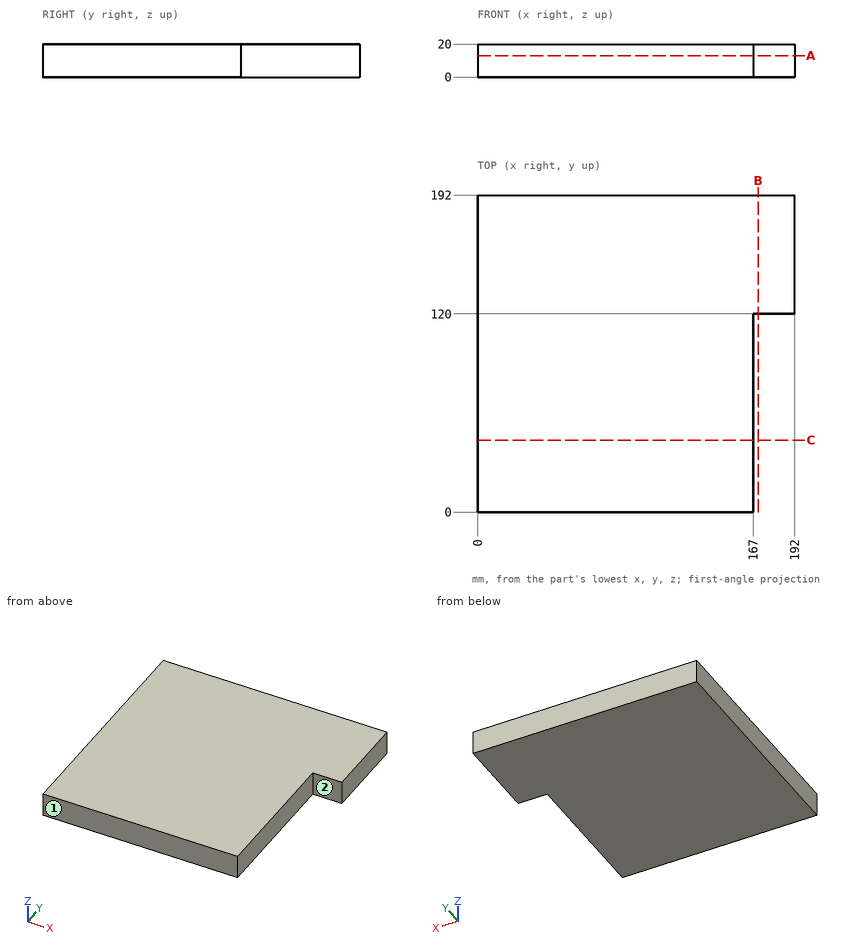
Geometry check sheet. Reference: drawing and pictorial views, mm from the part's lowest x, y, z. A direction names the side the tool comes from. Coordinates: 2 decimals unless noted, no trailing zeros. Loops run counter-clockwise (first coordinate to the right, second up) from the corner with the lowest first, then second, coordinate; pieces in that order, holes last.
1) Sectioned sample at A-A (z = 13). Record the boundary of the cut face in (x, y).
2) Gauge pin test, flat ends, axial feed: pin 1 (4 mm diameter, centred on y = 46.5, z = 8.5, fed in from -X); pin 2 (8 mm diameter, centred on y = 51.5, z = 17, fed in from +X). Record the tip position at first contact, or that the pin passes through.
3) Sectioned sample at C-C (y = 43.5). Record the boundary of the cut face in (x, z).
4) Sectioned sample at B-B (x = 170). Record the boundary of the cut face in (y, z), and give its area (3 significant figures).
5) Access from +Z, -Z, +X, -X, +Y, -Y to the whole of each face (thin tool, end or side, straight path). Record for the marked faces 1 and 2.
6) Material ranges on probe 1 along X at (y, z) = (106, 2), recorded low to high.
Check sheet entries:
1. outline: (0, 0) - (167, 0) - (167, 120) - (192, 120) - (192, 192) - (0, 192) - close
2. pin 1: stops at x = 0
2. pin 2: stops at x = 167
3. outline: (0, 0) - (167, 0) - (167, 20) - (0, 20) - close
4. outline: (120, 0) - (192, 0) - (192, 20) - (120, 20) - close
4. area: 1,440 mm2
5. face 1: +Z, -Z, +X, -X, -Y
5. face 2: +Z, -Z, +X, -Y
6. probe 1: x = 0 to 167
